from build123d import *

# Parameters (mm, degrees)
BOSS_EXTRUDE1_DEPTH      = 0.25
BOSS_EXTRUDE1_DEPTH_BACK = 1.7
SKETCH1_W                = 27.24
SKETCH1_H                = 52.24
SKETCH1_W_2              = 24.24
SKETCH1_H_2              = 49.24
SKETCH2_W                = 27.24
SKETCH2_H                = 52.24
SKETCH2_W_2              = 24.24
SKETCH2_H_2              = 34.18
BOSS_EXTRUDE2_DEPTH      = 1
SKETCH3_W                = 3
SKETCH3_H                = 34.18
BOSS_EXTRUDE3_DEPTH      = 1
SKETCH4_W                = 6
SKETCH4_H                = 34.18
CUT_EXTRUDE1_DEPTH       = 2.95
SKETCH5_W                = 3
SKETCH5_H                = 0.2
BOSS_EXTRUDE4_DEPTH      = 0.5
BOSS_EXTRUDE5_DEPTH      = 0.6
FILLET1_R                = 1
SKETCH8_W                = 16.74
SKETCH8_H                = 34.18
BOSS_EXTRUDE6_DEPTH      = 3.7
SKETCH7_R                = 1.65
CUT_EXTRUDE2_DEPTH       = 4.7
SKETCH10_R               = 3
CUT_EXTRUDE3_DEPTH       = 1.25
SKETCH12_W               = 6.25
SKETCH12_H               = 34.18
SKETCH12_W_2             = 7.24
BOSS_EXTRUDE7_DEPTH      = 4.7
SKETCH18_W               = 7.24
SKETCH18_H               = 34.18
CUT_EXTRUDE6_DEPTH       = 4.7
SKETCH19_W               = 1.5
SKETCH19_H               = 7.25
BOSS_EXTRUDE8_DEPTH      = 34.18
SKETCH20_W               = 6.25
SKETCH20_H               = 34.18
CUT_EXTRUDE7_DEPTH       = 4.7


with BuildPart() as part:
    # Sketch1 → Boss-Extrude1 (new, two sides: drawn at the far end of the back side and taken through both)
    with BuildSketch(Plane.XY.offset(-BOSS_EXTRUDE1_DEPTH_BACK)):
        Rectangle(SKETCH1_W, SKETCH1_H)
        Rectangle(SKETCH1_W_2, SKETCH1_H_2, mode=Mode.SUBTRACT)
    extrude(amount=BOSS_EXTRUDE1_DEPTH + BOSS_EXTRUDE1_DEPTH_BACK)

    # Sketch2 → Boss-Extrude2 (add)
    with BuildSketch(Plane.XY.offset(0.25)):
        Rectangle(SKETCH2_W, SKETCH2_H)
        Rectangle(SKETCH2_W_2, SKETCH2_H_2, mode=Mode.SUBTRACT)
    extrude(amount=BOSS_EXTRUDE2_DEPTH)

    # Sketch3 → Boss-Extrude3 (add)
    with BuildSketch(Plane.XY.offset(1.25)):
        with Locations((-6.12, 0)):
            Rectangle(SKETCH3_W, SKETCH3_H)
    extrude(amount=-BOSS_EXTRUDE3_DEPTH)

    # Sketch4 → Cut-Extrude1 (cut)
    with BuildSketch(Plane.XY.offset(1.25)):
        with Locations((-10.62, 0)):
            Rectangle(SKETCH4_W, SKETCH4_H)
    extrude(amount=-CUT_EXTRUDE1_DEPTH, mode=Mode.SUBTRACT)

    # Sketch5 → Boss-Extrude4 (add)
    with BuildSketch(Plane.XZ.offset(-24.62)):
        with Locations((0, -1.6)):
            Rectangle(SKETCH5_W, SKETCH5_H)
    boss_extrude4 = extrude(amount=BOSS_EXTRUDE4_DEPTH)

    # Mirror1: Boss-Extrude4 across plane
    add(boss_extrude4.mirror(Plane.ZX))

    # Sketch6 → Boss-Extrude5 (add)
    with BuildSketch(Plane(origin=(0, 0, -1.7), x_dir=(-1, 0, 0), z_dir=(0, 0, -1))):
        Polygon((13.62, -26.12), (13.62, -17.09), (12.12, -17.09), (12.12, -24.62), (1.5, -24.62), (1.5, -24.12), (-1.5, -24.12), (-1.5, -24.62), (-12.12, -24.62), (-12.12, 24.62), (-1.5, 24.62), (-1.5, 24.12), (1.5, 24.12), (1.5, 24.62), (12.12, 24.62), (12.12, 17.09), (13.62, 17.09), (13.62, 26.12), (-13.62, 26.12), (-13.62, -26.12), align=None)
    extrude(amount=BOSS_EXTRUDE5_DEPTH)

    # Fillet1
    # the kernel refuses this fillet: 1 mm, written as the material it adds along each edge
    with BuildSketch(Plane(origin=(1.5, -24.62, -2.3), x_dir=(1, 0, 0), z_dir=(0, 0, 1)), Plane(origin=(-1.5, -24.62, -1.5), x_dir=(-1, 0, 0), z_dir=(0, 0, -1)), Plane(origin=(1.5, 24.62, -1.5), x_dir=(1, 0, 0), z_dir=(0, 0, -1)), Plane(origin=(-1.5, 24.62, -2.3), x_dir=(-1, 0, 0), z_dir=(0, 0, 1))) as fillet1_piece_1:
        with BuildLine():
            CenterArc((0.866025404, 1), FILLET1_R, 210, 60)
            Line((0, 0.5), (-0.017320508, 0.49))
            ThreePointArc((-0.017320508, 0.49), (-0.02, 0.25), (-0.02, 0))
            Line((-0.02, 0), (0, -0.02))
            Line((0, -0.02), (0.866025404, -0.02))
            Line((0.866025404, -0.02), (0.866025404, 0))
        make_face()
    extrude(amount=0.8)

    # Sketch8 → Boss-Extrude6 (add)
    with BuildSketch(Plane.XY.offset(1.25)):
        Polygon((-7.62, -17.09), (-13.62, -17.09), (-13.62, -26.12), (13.62, -26.12), (13.62, 26.12), (-13.62, 26.12), (-13.62, 17.09), (-7.62, 17.09), align=None)
        with Locations((3.75, 0)):
            Rectangle(SKETCH8_W, SKETCH8_H, mode=Mode.SUBTRACT)
    extrude(amount=BOSS_EXTRUDE6_DEPTH)

    # Sketch7 → Cut-Extrude2 (cut)
    with BuildSketch(Plane(origin=(0, 0, 0.25), x_dir=(-1, 0, 0), z_dir=(0, 0, -1))):
        with Locations((0, 21.59)):
            Circle(SKETCH7_R)
        with Locations((0, -21.59)):
            Circle(SKETCH7_R)
    extrude(amount=-CUT_EXTRUDE2_DEPTH, mode=Mode.SUBTRACT)

    # Sketch10 → Cut-Extrude3 (cut)
    with BuildSketch(Plane.XY.offset(4.95)):
        with Locations((0, 21.59)):
            Circle(SKETCH10_R)
        with Locations(Location((0, -21.59, 0), (0, 0, 180))):
            Circle(SKETCH10_R)
    extrude(amount=-CUT_EXTRUDE3_DEPTH, mode=Mode.SUBTRACT)

    # Sketch12 → Boss-Extrude7 (add)
    with BuildSketch(Plane(origin=(0, 0, 0.25), x_dir=(-1, 0, 0), z_dir=(0, 0, -1))):
        with Locations((-8.995, 0)):
            Rectangle(SKETCH12_W, SKETCH12_H)
        with Locations((6.25, 0)):
            Rectangle(SKETCH12_W_2, SKETCH12_H)
    extrude(amount=-BOSS_EXTRUDE7_DEPTH)

    # Sketch18 → Cut-Extrude6 (cut)
    with BuildSketch(Plane(origin=(0, 0, 0.25), x_dir=(-1, 0, 0), z_dir=(0, 0, -1))):
        with Locations((6.25, 0)):
            Rectangle(SKETCH18_W, SKETCH18_H)
    extrude(amount=-CUT_EXTRUDE6_DEPTH, mode=Mode.SUBTRACT)

    # Sketch19 → Boss-Extrude8 (add)
    with BuildSketch(Plane(origin=(0, -17.09, 0), x_dir=(1, 0, 0), z_dir=(0, 1, 0))):
        with Locations((-12.87, -1.325)):
            Rectangle(SKETCH19_W, SKETCH19_H)
    extrude(amount=BOSS_EXTRUDE8_DEPTH)

    # Sketch20 → Cut-Extrude7 (cut)
    with BuildSketch(Plane(origin=(0, 0, 0.25), x_dir=(-1, 0, 0), z_dir=(0, 0, -1))):
        with Locations((-8.995, 0)):
            Rectangle(SKETCH20_W, SKETCH20_H)
    extrude(amount=-CUT_EXTRUDE7_DEPTH, mode=Mode.SUBTRACT)


solid = part.part
For this review, take the finished solid that the model builds, in its own axes (mm). A direction names the side the tool comes from. Give positions to 0.01 mm unless a question says otherwise; leave off trailing zeros. Loops run counter-clockwise (first coordinate to the right, second up) from the corner with the lowest first, then second, coordinate; pieces in that order, holes last. Notation, with made-up numbers: (5.5, 20.5) -> (45.5, 20.5) arc R14 cw to (45.5, 27.5) -> close; hole circle Ø4 at (-36.5, -20.5). An arc over 180 degrees is marked (long way). One line per question, with ' | ' between items.
1) We need section C-C (y = 2). Write out the cut boundary in (x, z).
Resolved:
outline: (-13.62, -2.3) -> (-12.12, -2.3) -> (-12.12, 4.95) -> (-13.62, 4.95) -> close; (12.12, -2.3) -> (13.62, -2.3) -> (13.62, 4.95) -> (12.12, 4.95) -> close
2) We need section D-D (x = 0). Give the number of separate pieces and of enclosed holes in the cut face, plus the area to 3 significant figures.
Resolved:
separate pieces: 4 | enclosed holes: 0 | area: 55.6 mm2
3) We need section A-A (z = 4.25). Write out the cut boundary in (x, y), plus the area to 3 significant figures.
Resolved:
outline: (-13.62, -26.12) -> (13.62, -26.12) -> (13.62, 26.12) -> (-13.62, 26.12) -> close; hole (-12.12, -17.09) -> (12.12, -17.09) -> (12.12, 17.09) -> (-12.12, 17.09) -> close; hole circle Ø6 at (0, -21.59); hole circle Ø6 at (0, 21.59) | area: 538 mm2
4) Insertion check: pin 1 Ø4 at (x, y) = (-4.5, 22) entering from -Z; pin 2 Ø5.5 at (x, y) = (0, 21.59) entering from +Z. Each pin has a flat end and moves straight along its axis. Give the tip position at first contact, or say it passes through.
Resolved:
pin 1: stops at z = 0.25 | pin 2: stops at z = 3.7
5) We need section B-B (x = -10.25). Write out the cut boundary in (y, z).
Resolved:
outline: (-26.12, -2.3) -> (-24.62, -2.3) -> (-24.62, 0.25) -> (-17.09, 0.25) -> (-17.09, 4.95) -> (-26.12, 4.95) -> close; (17.09, 0.25) -> (24.62, 0.25) -> (24.62, -2.3) -> (26.12, -2.3) -> (26.12, 4.95) -> (17.09, 4.95) -> close
6) To check wall thickness, follow probe 1 along Y at (x, z) = (0, 4.1); probe 2 along Y at (x, z) = (0, 1.05); probe 3 along X at (y, z) = (-21.59, 4.55). State the ranges of each line that lie inside material, in increasing order.
Resolved:
probe 1: y = -26.12 to -24.59, -18.59 to -17.09, 17.09 to 18.59, 24.59 to 26.12 | probe 2: y = -26.12 to -23.24, -19.94 to -17.09, 17.09 to 19.94, 23.24 to 26.12 | probe 3: x = -13.62 to -3, 3 to 13.62
7) For faces 4 (the flat face through (0, 17.09, 3)), 5 (the flat face through (1, 20, 3.7)), 6 (the flat face through (-13.62, 0, 1)), list the 3-axis set-ups (+Z, -Z, +X, -X, +Y, -Y) from which the entire face can be reached by the end or side of a thin tool; tool diameter is ignored.
Resolved:
face 4: +Z, -Z | face 5: +Z | face 6: +Z, -Z, -X, +Y, -Y
8) The part is to be moulded in two halves that separate along Y. For faces 1 (the flat face through (0, 26.12, 1)), 2 (the flat face through (-13, 2, -2.3)), 3 (the flat face through (-1, -20, 3.7)), say which applies: +Y half, -Y half, draft (parallel to the pull), parting line (faces both ways), or undercut.
Resolved:
face 1: +Y half | face 2: draft | face 3: undercut
